The model under review builds one solid part; all positions refer to its coordinate system, in mm. A direction names the side the tool comes from. Round coordinates to 2 decimals unless told otherwise and drop trailing zeros. Loops run counter-clockwise (first coordinate to the right, second up) from the corner with the lowest first, then second, coordinate; pieces in that order, holes last. Notation, with made-up numbers: (22, 78) -> (50, 78) arc R14 cw to (50, 85) -> close; hole circle Ø8 at (-13.5, -21). An arc over 180 degrees is marked (long way). Use a Markdown table: item, result. Add a question column.
1) Wall thickness on probe 1 along Y at (x, z) = (-63, 0.25); probe 2 along X at (y, z) = (-5, -1.5); probe 3 along Y at (x, z) = (-63, -1.5): over which ranges is each line inside the solid? List them lowest first.
2) Consider section A-A on y = 0. Give the boundary of the cut face in (x, z), plus the area to 3 significant figures.
3) Consider section C-C on x = -43.5. Give the boundary of the cut face in (y, z).
4) For faces 1 (the cylindrical face through (-64.51, -4.88, 1.08)), 2 (the cylindrical face through (40.84, -4.88, 1.08)), 3 (the flat face through (-100, 0, 0)), list the 3-axis set-ups (+Z, -Z, +X, -X, +Y, -Y) from which the entire face can be reached by the end or side of a thin tool; tool diameter is ignored.
5) Insertion check: pin 1 (4 mm diameter, centred on x = 35, y = 1, fed in from -Z); pin 2 (1 mm diameter, centred on x = 6.5, y = -4, fed in from +Z); pin 3 (6 mm diameter, centred on x = 79, z = 1, fed in from -Y). Each pin has a flat end and moves straight along its axis. Give the tip position at first contact, or say it passes through.
from build123d import *

# Parameters (mm, degrees)
SKETCH1_R           = 5
BOSS_EXTRUDE1_DEPTH = 100
BOSS_EXTRUDE2_START = -70
SKETCH2_R           = 7
BOSS_EXTRUDE2_DEPTH = 10


with BuildPart() as part:
    # Sketch1 → Boss-Extrude1 (new body, symmetric)
    with BuildSketch(Plane(origin=(0, 0, 0), x_dir=(0, 0, -1), z_dir=(1, 0, 0))):
        Circle(SKETCH1_R)
    extrude(amount=BOSS_EXTRUDE1_DEPTH, both=True)

    # Sketch2 → Boss-Extrude2 (add)
    with BuildSketch(Plane.ZY.offset(100).offset(BOSS_EXTRUDE2_START)):
        Circle(SKETCH2_R)
    extrude(amount=-BOSS_EXTRUDE2_DEPTH)


solid = part.part
Result set:
| question | item | result |
|---|---|---|
| 1 | probe 1 | -4.99 to 4.99 |
| 1 | probe 2 | -30 to -20 |
| 1 | probe 3 | -4.77 to 4.77 |
| 2 | outline | (-100, -5) -> (-30, -5) -> (-30, -7) -> (-20, -7) -> (-20, -5) -> (100, -5) -> (100, 5) -> (-20, 5) -> (-20, 7) -> (-30, 7) -> (-30, 5) -> (-100, 5) -> close |
| 2 | area | 2,040 mm2 |
| 3 | outline | circle Ø10 at (0, 0) |
| 4 | face 1 | -X |
| 4 | face 2 | +X |
| 4 | face 3 | +Z, -Z, -X, +Y, -Y |
| 5 | pin 1 | z = -5 |
| 5 | pin 2 | z = 3.57 |
| 5 | pin 3 | y = -5 |
